Source: CAD feature listing. Evaluate the final solid. Frame: model axes, mm. A direction names the side the tool comes from. Give positions to 0.01 mm unless a question says otherwise; leave off trailing zeros. Order: outer loops, then holes, each group sorted by start corner. A loop starts at its lowest first (then second) coordinate and runs counter-clockwise, first axis right, second up.
```python
from build123d import *

# Parameters (mm, degrees)
SKETCH1_W           = 45
SKETCH1_H           = 65
BOSS_EXTRUDE1_DEPTH = 40
SKETCH2_W           = 12.75
SKETCH2_H           = 3
CUT_EXTRUDE1_DEPTH  = 40
CUT_EXTRUDE2_DEPTH  = 7.5
CUT_EXTRUDE3_DEPTH  = 18.5
SKETCH6_W           = 13
SKETCH6_H           = 23
CUT_EXTRUDE4_DEPTH  = 1.5
SKETCH7_R           = 9.5
CUT_EXTRUDE5_DEPTH  = 11
SKETCH8_R           = 1
CUT_EXTRUDE6_DEPTH  = 10
FILLET1_R           = 2.5
FILLET2_R           = 2.5
FILLET3_R           = 2.5
FILLET4_R           = 1
FILLET5_R           = 9.5


# Some blends are built 0.0001 mm under size
with BuildPart() as part:
    # Sketch1 → Boss-Extrude1 (new body)
    with BuildSketch(Plane(origin=(0, 0, 0), x_dir=(1, 0, 0), z_dir=(0, 1, 0))):
        Rectangle(SKETCH1_W, SKETCH1_H)
    extrude(amount=BOSS_EXTRUDE1_DEPTH)

    # Sketch2 → Cut-Extrude1 (cut)
    with BuildSketch(Plane(origin=(0, 40, 0), x_dir=(1, 0, 0), z_dir=(0, 1, 0))):
        with Locations((-16.125, 31)):
            Rectangle(SKETCH2_W, SKETCH2_H)
        with Locations((16.125, 31)):
            Rectangle(SKETCH2_W, SKETCH2_H)
        with Locations((-16.125, -31)):
            Rectangle(SKETCH2_W, SKETCH2_H)
        with Locations((16.125, -31)):
            Rectangle(SKETCH2_W, SKETCH2_H)
    extrude(amount=-CUT_EXTRUDE1_DEPTH, mode=Mode.SUBTRACT)

    # Sketch3 → Cut-Extrude2 (cut)
    with BuildSketch(Plane(origin=(0, 40, 0), x_dir=(1, 0, 0), z_dir=(0, 1, 0))):
        Polygon((-22.5, 29.5), (-9.75, 29.5), (-9.75, 18.5), (-12, 18.5), (-12, -18.5), (-9.75, -18.5), (-9.75, -29.5), (-22.5, -29.5), (-22.5, -18.5), (-22.5, 18.5), align=None)
        Polygon((22.5, -29.5), (9.75, -29.5), (9.75, -18.5), (12, -18.5), (12, 18.5), (9.75, 18.5), (9.75, 29.5), (22.5, 29.5), (22.5, 18.5), (22.5, -18.5), align=None)
    extrude(amount=-CUT_EXTRUDE2_DEPTH, mode=Mode.SUBTRACT)

    # Sketch5 → Cut-Extrude3 (cut)
    with BuildSketch(Plane(origin=(0, 40, 0), x_dir=(1, 0, 0), z_dir=(0, 1, 0))):
        Polygon((-20, 29.5), (-12, 29.5), (-9.75, 29.5), (-9.75, 18.5), (-12, 18.5), (-12, -18.5), (-9.75, -18.5), (-9.75, -29.5), (-12, -29.5), (-20, -29.5), align=None)
        Polygon((12, -29.5), (9.75, -29.5), (9.75, -18.5), (12, -18.5), (12, 18.5), (9.75, 18.5), (9.75, 29.5), (12, 29.5), (20, 29.5), (20, -29.5), align=None)
    extrude(amount=-CUT_EXTRUDE3_DEPTH, mode=Mode.SUBTRACT)

    # Sketch6 → Cut-Extrude4 (cut)
    with BuildSketch(Plane(origin=(0, 40, 0), x_dir=(1, 0, 0), z_dir=(0, 1, 0))):
        with Locations((0, 35)):
            Rectangle(SKETCH6_W, SKETCH6_H)
        with Locations((0, -35)):
            Rectangle(SKETCH6_W, SKETCH6_H)
    extrude(amount=-CUT_EXTRUDE4_DEPTH, mode=Mode.SUBTRACT)

    # Sketch7 → Cut-Extrude5 (cut)
    with BuildSketch(Plane(origin=(0, 40, 0), x_dir=(1, 0, 0), z_dir=(0, 1, 0))):
        with Locations(Location((0, -12, 0), (0, 0, 270))):
            Circle(SKETCH7_R)
        with Locations(Location((0, 12, 0), (0, 0, 90))):
            Circle(SKETCH7_R)
    extrude(amount=-CUT_EXTRUDE5_DEPTH, mode=Mode.SUBTRACT)

    # Sketch8 → Cut-Extrude6 (cut)
    with BuildSketch(Plane(origin=(0, 21.5, 0), x_dir=(1, 0, 0), z_dir=(0, 1, 0))):
        with Locations(Location((-16, 20, 0), (0, 0, 270))):
            Circle(SKETCH8_R)
        with Locations(Location((16, 20, 0), (0, 0, 270))):
            Circle(SKETCH8_R)
        with Locations(Location((16, -20, 0), (0, 0, 270))):
            Circle(SKETCH8_R)
        with Locations(Location((-16, -20, 0), (0, 0, 270))):
            Circle(SKETCH8_R)
    extrude(amount=-CUT_EXTRUDE6_DEPTH, mode=Mode.SUBTRACT)

    # Fillet1
    fillet1_edges = [part.edges().sort_by_distance(p)[0] for p in [
        (-20, 32.5, 0),
    ]]
    fillet(fillet1_edges, radius=FILLET1_R - 0.0001)  # a hair under: the kernel refuses the full size

    # Fillet2
    fillet2_edges = [part.edges().sort_by_distance(p)[0] for p in [
        (20, 32.5, 0),
    ]]
    fillet(fillet2_edges, radius=FILLET2_R - 0.0001)  # a hair under: the kernel refuses the full size

    # Fillet3
    fillet3_edges = [part.edges().sort_by_distance(p)[0] for p in [
        (9.75, 20, -32.5),
        (-9.75, 20, 32.5),
        (-9.75, 20, -32.5),
        (9.75, 20, 32.5),
    ]]
    fillet(fillet3_edges, radius=FILLET3_R)

    # Fillet4
    fillet4_edges = [part.edges().sort_by_distance(p)[0] for p in [
        (22.5, 16.25, -29.5),
        (-22.5, 16.25, 29.5),
        (-22.5, 16.25, -29.5),
        (22.5, 16.25, 29.5),
    ]]
    fillet(fillet4_edges, radius=FILLET4_R)

    # Fillet5
    # the kernel refuses this fillet: 9.5 mm, written as the material it takes off along each edge
    with BuildSketch(Plane(origin=(12, 55.347536447, 18.5), x_dir=(-1, 0, 0), z_dir=(0, -1, 0)), Plane(origin=(-12, 55.347536447, -18.5), x_dir=(1, 0, 0), z_dir=(0, -1, 0))) as fillet5_piece_1:
        with BuildLine():
            CenterArc((9.5, 6.139014579), FILLET5_R, 180, 40.256612576)
            Line((0, 6.139014579), (-0.19, 6.139014579))
            Line((-0.19, 6.139014579), (-0.19, 0))
            Line((-0.19, 0), (0, -0.19))
            ThreePointArc((0, -0.19), (1.125, -0.19), (2.105, -0.122780292))
            Line((2.105, -0.122780292), (2.25, 0))
        make_face()
    extrude(amount=33.847536447, mode=Mode.SUBTRACT)
    with BuildSketch(Plane(origin=(-12, 55.347536447, 18.5), x_dir=(1, 0, 0), z_dir=(0, -1, 0)), Plane(origin=(12, 55.347536447, -18.5), x_dir=(-1, 0, 0), z_dir=(0, -1, 0))) as fillet5_piece_2:
        with BuildLine():
            CenterArc((9.5, -6.139014579), FILLET5_R, 139.743387424, 40.256612576)
            Line((0, -6.139014579), (-0.19, -6.139014579))
            Line((-0.19, -6.139014579), (-0.19, 0))
            Line((-0.19, 0), (0, 0.19))
            ThreePointArc((0, 0.19), (1.125, 0.19), (2.105, 0.122780292))
            Line((2.105, 0.122780292), (2.25, 0))
        make_face()
    extrude(amount=33.847536447, mode=Mode.SUBTRACT)


solid = part.part
```
1) Reachability of faces 4 (the flat face through (-9.75, 34, 24)), 5 (the cylindrical face through (-11.436, 30.88, -15.586)), 6 (the cylindrical face through (3.639, 34.577, -20.776)) from +Z, -Z, +X, -X, +Y, -Y: full face, straight path, thin tool, end or side. Return the list, or none.
Report:
face 4: +Z, +Y
face 5: -Z, +Y
face 6: +Y
2) Section query B-B, the plane y = 34.5. Return the cut outline in (x, z).
Report:
outline: (-12, -12.36) arc R9.5 ccw to (-9.75, -18.5) - (-9.75, -30) arc R2.5 ccw to (-7.25, -32.5) - (7.25, -32.5) arc R2.5 ccw to (9.75, -30) - (9.75, -18.5) arc R9.5 ccw to (12, -12.36) - (12, 12.36) arc R9.5 ccw to (9.75, 18.5) - (9.75, 30) arc R2.5 ccw to (7.25, 32.5) - (-7.25, 32.5) arc R2.5 ccw to (-9.75, 30) - (-9.75, 18.5) arc R9.5 ccw to (-12, 12.36) - close; hole circle Ø19 at (0, -12); hole circle Ø19 at (0, 12)
3) Pin query (flat end, axial travel): pin 1 (1 mm diameter, centred on x = 16.5, z = -19.5, fed in from +Y); pin 2 (4.5 mm diameter, centred on x = 0, z = -30, fed in from +Y); pin 3 (1 mm diameter, centred on x = 16, y = 5, fed in from +Z). Return the tip coordinate at first contact, or that it passes through.
Report:
pin 1: stops at y = 21.5
pin 2: stops at y = 38.5
pin 3: stops at z = 29.5
4) Section query C-C, the plane x = 0. Return the cut outline in (y, z).
Report:
outline: (0, -32.5) - (38.5, -32.5) - (38.5, -23.5) - (40, -23.5) - (40, -21.5) - (29, -21.5) - (29, -2.5) - (40, -2.5) - (40, 2.5) - (29, 2.5) - (29, 21.5) - (40, 21.5) - (40, 23.5) - (38.5, 23.5) - (38.5, 32.5) - (0, 32.5) - close
5) Section query D-D, the plane y = 4.5. Return the cut outline in (x, z), and give its area (3 significant figures).
Report:
outline: (-22.5, -28.5) arc R1 ccw to (-21.5, -29.5) - (-9.75, -29.5) - (-9.75, -30) arc R2.5 ccw to (-7.25, -32.5) - (7.25, -32.5) arc R2.5 ccw to (9.75, -30) - (9.75, -29.5) - (21.5, -29.5) arc R1 ccw to (22.5, -28.5) - (22.5, 28.5) arc R1 ccw to (21.5, 29.5) - (9.75, 29.5) - (9.75, 30) arc R2.5 ccw to (7.25, 32.5) - (-7.25, 32.5) arc R2.5 ccw to (-9.75, 30) - (-9.75, 29.5) - (-21.5, 29.5) arc R1 ccw to (-22.5, 28.5) - close
area: 2,770 mm2
6) Material intervals for L1, parallel to X at y = 15.25, z = -20; L2, parallel to X at y = 28.5, z = -20.5; L3, parallel to Z at x = 1, y = 33.5, sorted ascending.
Report:
L1: x = -22.5 to -17, -15 to 15, 17 to 22.5
L2: x = -22.5 to -20, -9.75 to 9.75, 20 to 22.5
L3: z = -32.5 to -21.45, -2.55 to 2.55, 21.45 to 32.5
7) Draft query along X for faces 1 (the flat face through (-16, 13, -29.5)), 2 (the flat face through (6.5, 39, -28)), 3 (the flat face through (22.5, 16, 0)). Return one class per face: +X half, -X half, draft (parallel to the pull), parting line (faces both ways), or undercut.
Report:
face 1: draft
face 2: undercut
face 3: +X half
8) Section query A-A, the plane y = 15. Return the cut outline in (x, z).
Report:
outline: (-22.5, -28.5) arc R1 ccw to (-21.5, -29.5) - (-9.75, -29.5) - (-9.75, -30) arc R2.5 ccw to (-7.25, -32.5) - (7.25, -32.5) arc R2.5 ccw to (9.75, -30) - (9.75, -29.5) - (21.5, -29.5) arc R1 ccw to (22.5, -28.5) - (22.5, 28.5) arc R1 ccw to (21.5, 29.5) - (9.75, 29.5) - (9.75, 30) arc R2.5 ccw to (7.25, 32.5) - (-7.25, 32.5) arc R2.5 ccw to (-9.75, 30) - (-9.75, 29.5) - (-21.5, 29.5) arc R1 ccw to (-22.5, 28.5) - close; hole circle Ø2 at (-16, -20); hole circle Ø2 at (-16, 20); hole circle Ø2 at (16, -20); hole circle Ø2 at (16, 20)
